Could you check a few things on this model? Use its own coordinates, in mm. A direction names the side the tool comes from. Give positions to 0.01 mm unless a question says otherwise; leave off trailing zeros. Write each loop counter-clockwise with the first axis right and the second up, starting at its lowest first coordinate (ties: lowest second). Pieces come first, ordered by that corner, then holes. Notation, with made-up numbers: (29, 11) -> (81, 11) arc R30 cw to (81, 33) -> close; hole circle Ø1 at (57, 75). An arc over 180 degrees is marked (long way). One line per question, with ' | ' between items.
from build123d import *

# Parameters (mm, degrees)
SKETCH001_W     = 45
SKETCH001_H     = 105
SKETCH001_R     = 3
PAD_DEPTH       = 2
SKETCH_R        = 3
PAD001_DEPTH    = 10
SKETCH004_W     = 7
SKETCH004_H     = 10
PAD003_DEPTH    = 45
POCKET001_DEPTH = 82.501
SKETCH006_R     = 2
POCKET002_DEPTH = 5


with BuildPart() as part:
    # Sketch001 → Pad (new body)
    with BuildSketch(Plane.XY.offset(10)):
        with Locations((-22.5, -6.5)):
            Rectangle(SKETCH001_W, SKETCH001_H)
        with Locations((-37.5, 40)):
            Circle(SKETCH001_R, mode=Mode.SUBTRACT)
        with Locations((-37.5, -35)):
            Circle(SKETCH001_R, mode=Mode.SUBTRACT)
        with BuildLine():
            ThreePointArc((-20.9, 32), (-22.9, 30), (-20.9, 28))
            Line((-20.9, 28), (-18.9, 28))
            ThreePointArc((-18.9, 28), (-16.9, 30), (-18.9, 32))
            Line((-20.9, 32), (-18.9, 32))
        make_face(mode=Mode.SUBTRACT)
        with BuildLine():
            ThreePointArc((-19.514425, -27.18234), (-22.332089, -27.428853), (-22.085575, -30.246517))
            Line((-22.085575, -30.246517), (-20.553491, -31.532089))
            ThreePointArc((-20.553491, -31.532089), (-17.735828, -31.285577), (-17.982336, -28.467915))
            Line((-19.514425, -27.18234), (-17.982336, -28.467915))
        make_face(mode=Mode.SUBTRACT)
    pad = extrude(amount=PAD_DEPTH)

    # Sketch (on Face16 of Pad) → Pad001 (join)
    with BuildSketch(Plane.XY.offset(12)):
        with Locations((-20, -23)):
            Circle(SKETCH_R)
        with Locations((-20, 23)):
            Circle(SKETCH_R)
    pad001 = extrude(amount=PAD001_DEPTH)

    # Mirrored: Pad across Sketch001 V_Axis
    add(pad.mirror(Plane(origin=(0, 0, 10), x_dir=(0, 0, 1), z_dir=(1, 0, 0))))

    # Mirrored001: Pad001 across Sketch V_Axis
    add(pad001.mirror(Plane(origin=(0, 0, 12), x_dir=(0, 0, 1), z_dir=(1, 0, 0))))

    # Sketch004 → Pad003 (join)
    with BuildSketch(Plane.XY.offset(12)):
        with Locations((34, -10)):
            Rectangle(SKETCH004_W, SKETCH004_H)
    extrude(amount=PAD003_DEPTH)

    # Sketch005 (on Face36 of Pad003) → Pocket001 (cut, through all)
    with BuildSketch(Plane(origin=(37.5, 0, 10), x_dir=(0, 1, 0), z_dir=(1, 0, 0))):
        Polygon((-7, 28.39), (-13, 28.39), (-13, 43.39), (-11.4, 45), (-8.6, 45), (-7, 43.39), align=None)
    extrude(amount=-POCKET001_DEPTH, mode=Mode.SUBTRACT)

    # Sketch006 (on Face42 of Pocket001) → Pocket002 (cut)
    with BuildSketch(Plane.XY.offset(57)):
        with Locations((34, -10)):
            Circle(SKETCH006_R)
    extrude(amount=-POCKET002_DEPTH, mode=Mode.SUBTRACT)


solid = part.part
Q1. On a 3-axis mill with a long thin cutter (end or side, diameter ignored), from which of +Z, -Z, +X, -X, +Y, -Y can I reach the whole of each face in a straight line? I mean faces 4 (the cylindrical face through (17.764, -31.319, 10.986)), 5 (the cylindrical face through (22.4, -24.8, 16.9)), 6 (the flat face through (34, -10, 38.39)). Say none if no direction works.
Answer below:
face 4: +Z, -Z | face 5: +Z | face 6: +X, -X
Q2. If we mould it in two halves opening along Y, with no side actions, what happens to faces 1 (the flat face through (20, 23, 22)), 2 (the flat face through (34, -5, 34)), 3 (the flat face through (34, -13, 46))? For each: +Y half, -Y half, draft (parallel to the pull), parting line (faces both ways), or undercut.
Answer below:
face 1: draft | face 2: +Y half | face 3: undercut
Q3. Imagine slicing it at C-C on z = 42. Please give me the cut outline in (x, y), and give its area (3 significant figures).
Answer below:
outline: (30.5, -15) -> (37.5, -15) -> (37.5, -13) -> (30.5, -13) -> close; (30.5, -7) -> (37.5, -7) -> (37.5, -5) -> (30.5, -5) -> close | area: 28.0 mm^2
Q4. Will these pins go through, and if not, where does the flat tip stop? pin 1 (3.5 mm diameter, centred on x = 34.5, z = 26, fed in from -Y); pin 2 (5 mm diameter, centred on x = -20, y = 23.5, fed in from +Z); pin 3 (5.5 mm diameter, centred on x = 35.5, z = 35.5, fed in from +Y).
Answer below:
pin 1: stops at y = -15 | pin 2: stops at z = 22 | pin 3: stops at y = -5
Q5. If I drill on line 1 along Y through (x, z) = (37.5, 10.45); line 2 along Y through (x, z) = (33.5, 41); line 3 along Z through (x, y) = (-17.5, -48), over which ranges is the centre line in solid material (lowest first)?
Answer below:
line 1: y = -59 to -38, -32 to 37, 43 to 46 | line 2: y = -15 to -13, -7 to -5 | line 3: z = 10 to 12
Q6. Imagine slicing it at B-B on y = -35. Please give me the cut outline in (x, z).
Answer below:
outline: (-45, 10) -> (-40.5, 10) -> (-40.5, 12) -> (-45, 12) -> close; (-34.5, 10) -> (34.5, 10) -> (34.5, 12) -> (-34.5, 12) -> close; (40.5, 10) -> (45, 10) -> (45, 12) -> (40.5, 12) -> close
Q7. Imagine slicing it at A-A on x = -37.5. Please give me the cut outline in (y, z).
Answer below:
outline: (-59, 10) -> (-38, 10) -> (-38, 12) -> (-59, 12) -> close; (-32, 10) -> (37, 10) -> (37, 12) -> (-32, 12) -> close; (43, 10) -> (46, 10) -> (46, 12) -> (43, 12) -> close
Q8. Imagine slicing it at D-D on y = -10. Please give me the cut outline in (x, z).
Answer below:
outline: (-45, 10) -> (45, 10) -> (45, 12) -> (37.5, 12) -> (37.5, 38.39) -> (30.5, 38.39) -> (30.5, 12) -> (-45, 12) -> close; (30.5, 55) -> (32, 55) -> (32, 57) -> (30.5, 57) -> close; (36, 55) -> (37.5, 55) -> (37.5, 57) -> (36, 57) -> close
